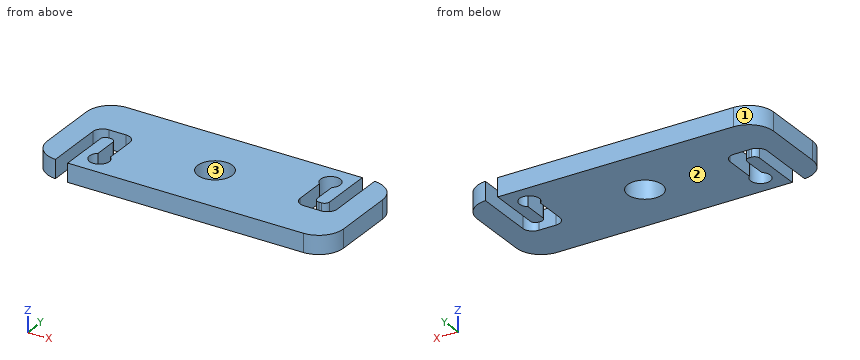
```python
from build123d import *

# Parameters (mm, degrees)
F1_DEPTH = 19.05
F2_R     = 17.78
F3_DEPTH = 19.051
F5_DEPTH = 19.051


with BuildPart() as f1:
    # F0 (on Top) → F1 (new body)
    with BuildSketch(Plane.XY):
        with BuildLine():
            ThreePointArc((152.4, 31.75), (144.9605122421, 49.7105122421), (127, 57.15))
            Line((127, 57.15), (-127, 57.15))
            ThreePointArc((-127, 57.15), (-144.9605122421, 49.7105122421), (-152.4, 31.75))
            Line((-152.4, 31.75), (-152.4, -31.75))
            ThreePointArc((-152.4, -31.75), (-144.9605122421, -49.7105122421), (-127, -57.15))
            Line((-127, -57.15), (127, -57.15))
            ThreePointArc((127, -57.15), (144.9605122421, -49.7105122421), (152.4, -31.75))
            Line((152.4, -31.75), (152.4, 31.75))
        make_face()
    extrude(amount=F1_DEPTH)

    # F2 (on face) → F3 (cut, through all)
    with BuildSketch(Plane.XY.offset(19.05)):
        Circle(F2_R)
    extrude(amount=-F3_DEPTH, mode=Mode.SUBTRACT)

    # F4 (on face) → F5 (cut, through all)
    with BuildSketch(Plane.XY.offset(19.05)):
        with BuildLine():
            Line((128.27, -3.81), (128.27, 57.15))
            Line((128.27, 57.15), (115.57, 57.15))
            Line((115.57, 57.15), (115.57, 3.81))
            ThreePointArc((115.57, 3.81), (114.0821024484, 0.2178975516), (110.49, -1.27))
            Line((110.49, -1.27), (107.95, -1.27))
            ThreePointArc((107.95, -1.27), (104.3578975516, 0.2178975516), (102.87, 3.81))
            Line((102.87, 3.81), (102.87, 27.628852542))
            ThreePointArc((102.87, 27.628852542), (96.52, 45.72), (90.17, 27.628852542))
            Line((90.17, 27.628852542), (90.17, -3.81))
            ThreePointArc((90.17, -3.81), (93.1457951031, -10.9942048969), (100.33, -13.97))
            Line((100.33, -13.97), (118.11, -13.97))
            ThreePointArc((118.11, -13.97), (125.2942048969, -10.9942048969), (128.27, -3.81))
        make_face()
        with BuildLine():
            Line((-128.27, 3.81), (-128.27, -57.1182301314))
            ThreePointArc((-128.27, -57.1182301314), (-127.6351986549, -57.1420562907), (-127, -57.15))
            Line((-127, -57.15), (-115.57, -57.15))
            Line((-115.57, -57.15), (-115.57, -3.81))
            ThreePointArc((-115.57, -3.81), (-114.0821024484, -0.2178975516), (-110.49, 1.27))
            Line((-110.49, 1.27), (-107.95, 1.27))
            ThreePointArc((-107.95, 1.27), (-104.3578975516, -0.2178975516), (-102.87, -3.81))
            Line((-102.87, -3.81), (-102.87, -27.628852542))
            ThreePointArc((-102.87, -27.628852542), (-96.52, -45.72), (-90.17, -27.628852542))
            Line((-90.17, -27.628852542), (-90.17, 3.81))
            ThreePointArc((-90.17, 3.81), (-93.1457951031, 10.9942048969), (-100.33, 13.97))
            Line((-100.33, 13.97), (-118.11, 13.97))
            ThreePointArc((-118.11, 13.97), (-125.2942048969, 10.9942048969), (-128.27, 3.81))
        make_face()
    extrude(amount=-F5_DEPTH, mode=Mode.SUBTRACT)


solid = f1.part
```
Part model, mm, in its own coordinate system. Face numbers are marked on the shaded views. Round coordinates to 2 decimals unless told otherwise and drop trailing zeros. Loops run counter-clockwise (first coordinate to the right, second up) from the corner with the lowest first, then second, coordinate; pieces in that order, holes last. Notation, with made-up numbers: (24, -3) -> (33, -3) arc R18 cw to (33, 17) -> close; hole circle Ø8 at (-9, -36.75). An arc over 180 degrees is marked (long way). Use one line per item in the form item = value. Start each with the question number.
Item 1: Band-saw the part on A-A (x = 0). List the corners of the cut face in (y, z).
Item 2: Band-saw the part on D-D (x = -96.52). List the corners of the cut face in (y, z), plus the area to 3 significant figures.
Item 3: Two-plate mould, pull along X, no slides. Class the marked faces 1, 2 and 3: released by +X, released by -X, zero draft, split by the parting line, or undercut.
Item 4: Band-saw the part on C-C (y = -35.56). List the corners of the cut face in (x, z).
Item 5: Drill centre lines: line 1 along X through (y, z) = (19, 11.25); line 2 along X through (y, z) = (-26, 11.75); line 3 along Y through (x, z) = (0, 5). Where is each one in solid material? Low to high.
Item 6: Drop flat-ended pins along their axis: pin 1 Ø1.5 at (y, z) = (-38.5, 16.5) entering from -X; pin 2 Ø18.5 at (x, y) = (96.52, 35.56) entering from -Z. Give the stop position or say it passes through.
Data:
q1.outline = (-57.15, 0) -> (-17.78, 0) -> (-17.78, 19.05) -> (-57.15, 19.05) -> close; (17.78, 0) -> (57.15, 0) -> (57.15, 19.05) -> (17.78, 19.05) -> close
q2.outline = (-57.15, 0) -> (-45.72, 0) -> (-45.72, 19.05) -> (-57.15, 19.05) -> close; (13.23, 0) -> (57.15, 0) -> (57.15, 19.05) -> (13.23, 19.05) -> close
q2.area = 1,050 mm^2
q3.face_1 = released by -X
q3.face_2 = zero draft
q3.face_3 = undercut
q4.outline = (-152.11, 0) -> (-128.27, 0) -> (-128.27, 19.05) -> (-152.11, 19.05) -> close; (-115.57, 0) -> (-106.68, 0) -> (-106.68, 19.05) -> (-115.57, 19.05) -> close; (-86.36, 0) -> (152.11, 0) -> (152.11, 19.05) -> (-86.36, 19.05) -> close
q5.line_1 = -152.4 to 90.17, 102.87 to 115.57, 128.27 to 152.4
q5.line_2 = -152.4 to -128.27, -115.57 to -102.87, -90.17 to 152.4
q5.line_3 = -57.15 to -17.78, 17.78 to 57.15
q6.pin_1 = -151.68
q6.pin_2 = through
